Here's the drawing with two shaded views (mm, measured from the low corner). I have some questions. Give positions to 0.01 mm unless a question says otherwise; leave off trailing zeros. Write each loop counter-clockwise with the first axis right and the second up, starting at its lowest first coordinate (ties: lowest second). Pieces come first, ordered by that corner, then holes.
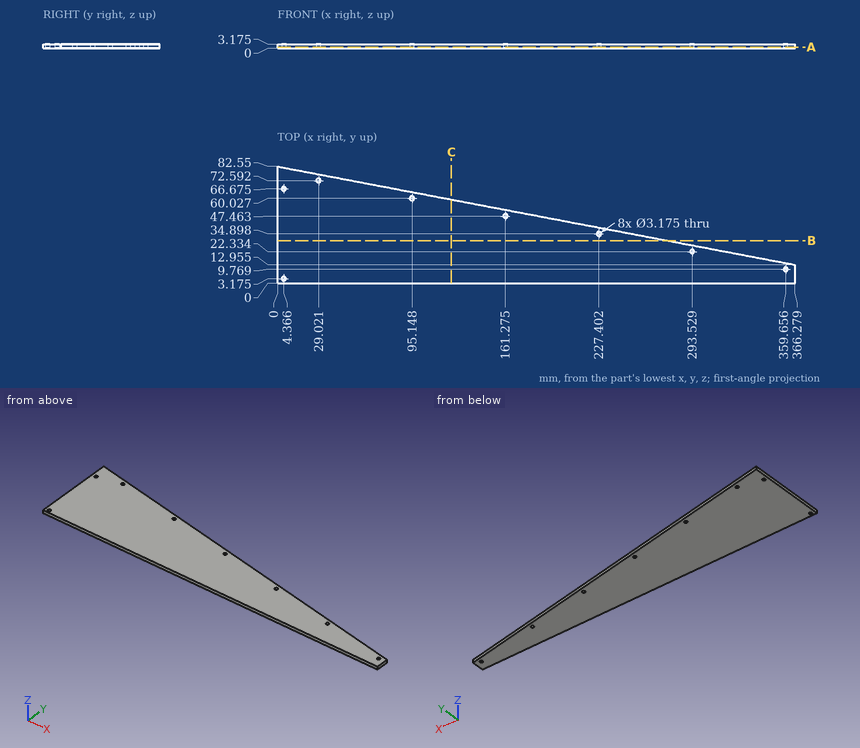
1) Please list where these lines run through material, in increasing order: L1, parallel to Y at x = 324, z = 1.1; L2, parallel to Y at x = 174, z = 1.95.
Values follow:
L1: y = 0 to 20.99
L2: y = 0 to 49.49
2) Suppose I cut it at C-C on x = 123. Write out the boundary of the cut face in (y, z) (1 decimal).
Values follow:
outline: (0, 0) - (59.2, 0) - (59.2, 3.2) - (0, 3.2) - close
3) Suppose I cut it at A-A on z = 0.95. State how many separate pieces and enclosed holes the cut face has, plus the area to 3 significant figures.
Values follow:
separate pieces: 1
enclosed holes: 8
area: 17,400 mm2
4) Suppose I cut it at B-B on y = 30. Write out the boundary of the cut face in (x, z) (1 decimal).
Values follow:
outline: (0, 0) - (276.6, 0) - (276.6, 3.2) - (0, 3.2) - close
